```python
from build123d import *

# Parameters (mm, degrees)
SKETCH2_W               = 7
SKETCH2_H               = 2.5
REVOLVE2_ANGLE          = 180
BOSS_EXTRUDE4_DEPTH     = 24
CUT_EXTRUDE1_DEPTH      = 3.5
SKETCH17_W              = 3
SKETCH17_H              = 5
CUT_EXTRUDE6_DEPTH      = 18
SKETCH16_R              = 1.52
CUT_EXTRUDE5_DEPTH      = 3.857492994
CUT_EXTRUDE5_DEPTH_BACK = 41.857492994
SKETCH19_R              = 2.02
CUT_EXTRUDE7_DEPTH      = 3
SKETCH20_R              = 2.02
CUT_EXTRUDE8_DEPTH      = 3
SKETCH21_R              = 15
CUT_EXTRUDE9_DEPTH      = 6.5
SKETCH22_R              = 5
BOSS_EXTRUDE6_DEPTH     = 6.5
SKETCH23_W              = 2
SKETCH23_H              = 3
SKETCH24_W              = 2
SKETCH24_H              = 3
SKETCH25_R              = 2
CUT_EXTRUDE11_DEPTH     = 20.5000001
SKETCH26_R              = 3.17
CUT_EXTRUDE12_DEPTH     = 6.5


with BuildPart() as part:
    # Sketch1 → Revolve1 (revolve)
    with BuildSketch(Plane.XY):
        Polygon((0, 0), (12, 10), (17, 10), (22, 10), (22, 8), (19, 8), (19, -7), (0, -7), align=None)
    revolve(axis=Axis((0, -7, 0), (0, 1, 0)))

    # Sketch2 → Revolve2 (revolve)
    with BuildSketch(Plane(origin=(0, 10, 0), x_dir=(1, 0, 0), z_dir=(0, 1, 0))):
        with Locations((15.5, 1.25)):
            Rectangle(SKETCH2_W, SKETCH2_H)
        with Locations((-15.5, 1.25)):
            Rectangle(SKETCH2_W, SKETCH2_H)
    revolve(axis=Axis((0, 10, 0), (1, 0, 0)), revolution_arc=REVOLVE2_ANGLE)

    # Sketch8 → Boss-Extrude4 (add)
    with BuildSketch(Plane(origin=(-12, 0, 0), x_dir=(0, 0, -1), z_dir=(1, 0, 0))):
        with BuildLine():
            Line((-2.5, 10), (0, 10))
            Line((0, 10), (2.5, 10))
            ThreePointArc((2.5, 10), (0, 12.5), (-2.5, 10))
        make_face()
    extrude(amount=BOSS_EXTRUDE4_DEPTH)

    # Sketch9 → Cut-Extrude1 (cut, through all)
    with BuildSketch(Plane(origin=(0, 10, 0), x_dir=(1, 0, 0), z_dir=(0, 1, 0))):
        with BuildLine():
            ThreePointArc((-11.736694594, 2.5), (-12, 0), (-11.736694594, -2.5))
            ThreePointArc((-11.736694594, -2.5), (0, -12), (11.736694594, -2.5))
            ThreePointArc((11.736694594, -2.5), (12, 0), (11.736694594, 2.5))
            ThreePointArc((11.736694594, 2.5), (0, 12), (-11.736694594, 2.5))
        make_face()
    extrude(amount=CUT_EXTRUDE1_DEPTH, mode=Mode.SUBTRACT)

    # Sketch17 → Cut-Extrude6 (cut, through all)
    with BuildSketch(Plane(origin=(0, 10, 0), x_dir=(1, 0, 0), z_dir=(0, 1, 0))):
        with Locations((20.5, 0)):
            Rectangle(SKETCH17_W, SKETCH17_H)
        with Locations((-20.5, 0)):
            Rectangle(SKETCH17_W, SKETCH17_H)
    extrude(amount=-CUT_EXTRUDE6_DEPTH, mode=Mode.SUBTRACT)

    # Sketch16 → Cut-Extrude5 (cut, two sides)
    with BuildSketch(Plane.ZY.offset(19)) as cut_extrude5_sk:
        with Locations((0, 10)):
            Circle(SKETCH16_R)
    extrude(amount=CUT_EXTRUDE5_DEPTH, mode=Mode.SUBTRACT)
    extrude(cut_extrude5_sk.sketch, amount=-CUT_EXTRUDE5_DEPTH_BACK, mode=Mode.SUBTRACT)

    # Sketch19 → Cut-Extrude7 (cut)
    with BuildSketch(Plane.ZY.offset(19)):
        with Locations((0, 10)):
            Circle(SKETCH19_R)
    extrude(amount=-CUT_EXTRUDE7_DEPTH, mode=Mode.SUBTRACT)

    # Sketch20 → Cut-Extrude8 (cut)
    with BuildSketch(Plane(origin=(19, 0, 0), x_dir=(0, 0, -1), z_dir=(1, 0, 0))):
        with Locations((0, 10)):
            Circle(SKETCH20_R)
    extrude(amount=-CUT_EXTRUDE8_DEPTH, mode=Mode.SUBTRACT)

    # Sketch21 → Cut-Extrude9 (cut)
    with BuildSketch(Plane.XZ.offset(7)):
        Circle(SKETCH21_R)
    extrude(amount=-CUT_EXTRUDE9_DEPTH, mode=Mode.SUBTRACT)

    # Sketch22 → Boss-Extrude6 (add)
    with BuildSketch(Plane.XZ.offset(0.5)):
        Circle(SKETCH22_R)
    extrude(amount=BOSS_EXTRUDE6_DEPTH)

    # Cut-Sweep2: sweep along a curve in space
    with BuildLine() as cut_sweep2_path:
        Line((10, -0.5, 0), (16, 8.48, 0))
        Line((16, 8.48, 0), (16.813206723, 9.697099395, 0))
    # Sketch23 → Cut-Sweep2 (sweep, cut)
    with BuildSketch(Plane.XZ.offset(0.5)):
        with Locations((11, 0)):
            Rectangle(SKETCH23_W, SKETCH23_H)
    sweep(path=cut_sweep2_path.line, mode=Mode.SUBTRACT)

    # Cut-Sweep3: sweep along a curve in space
    with BuildLine() as cut_sweep3_path:
        Line((-10, -0.5, 0), (-16, 8.48, 0))
        Line((-16, 8.48, 0), (-16.813206723, 9.697099395, 0))
    # Sketch24 → Cut-Sweep3 (sweep, cut)
    with BuildSketch(Plane.XZ.offset(0.5)):
        with Locations((-11, 0)):
            Rectangle(SKETCH24_W, SKETCH24_H)
    sweep(path=cut_sweep3_path.line, mode=Mode.SUBTRACT)

    # Sketch25 → Cut-Extrude11 (cut, through all)
    with BuildSketch(Plane.XZ.offset(7)):
        Circle(SKETCH25_R)
    extrude(amount=-CUT_EXTRUDE11_DEPTH, mode=Mode.SUBTRACT)

    # Sketch26 → Cut-Extrude12 (cut)
    with BuildSketch(Plane.XZ.offset(7)):
        Circle(SKETCH26_R)
    extrude(amount=-CUT_EXTRUDE12_DEPTH, mode=Mode.SUBTRACT)


solid = part.part
```
Can you work these out from the model? Positions are in its coordinate system, mm. A direction names the side the tool comes from. Coordinates: 2 decimals unless noted, no trailing zeros. Order: outer loops, then holes, each group sorted by start corner. A loop starts at its lowest first (then second) coordinate and runs counter-clockwise, first axis right, second up.
1. If we section it at C-C (y = 5.25): Please give me the cut outline in (x, z), then the cut area to 3 significant figures.
2. Thinking about a two-plate mould opening in Z: for faces 1 (the face through (1.5, 8, 19.1)), 2 (the face through (0, 9, -22)), 3 (the face through (-19, 12, 1)), which applies, +Z half, -Z half, draft (parallel to the pull), parting line (faces both ways), or undercut?
3. If we section it at A-A (x = 0): Please give me the cut outline in (y, z).
4. I need wall thicknesses on line 1 (Z direction, x = 0, y = -2.25); line 2 (Y direction, x = 18.4, z = 0); line 3 (Y direction, x = 14.1, z = 0). Which ranges of each line are inside material? Lowest first, please.
5. I'm going to push flat-ended pins straight in: pin 1 (15.5 mm diameter, centred on x = 10, z = -11, fed in from +Y); pin 2 (8 mm diameter, centred on y = 2.5, z = -15.5, fed in from -X); pin 3 (1.9 mm diameter, centred on x = 0.5, z = 1.5, fed in from -Y); pin 4 (4 mm diameter, centred on x = -3.5, z = 13, fed in from -Y). Where does each tip first touch, or does it pass through?
6. If we section it at D-D (x = -14): Please give me the cut outline in (y, z).
7. If we section it at B-B (z = 13.5): Please give me the cut outline in (x, y).
8. For faces 4 (the face through (17.521, 12.003, 0.263)), 5 (the face through (20, 9, -2.5)), 6 (the face through (14, 4, -1.5)), 7 (the face through (1.5, 8, -19.2)), 8 (the face through (-2.516, -3.796, -1.929)), which set-ups out of +Z, -Z, +X, -X, +Y, -Y let a thin tool reach every point of the face, with its end or its side?
Entries:
1. outline: circle Ø38 at (0, 0); hole (-15.84, -1.5) - (-13.84, -1.5) - (-13.84, 1.5) - (-15.84, 1.5) - close; hole circle Ø12.6 at (0, 0); hole (13.84, -1.5) - (15.84, -1.5) - (15.84, 1.5) - (13.84, 1.5) - close
1. area: 997 mm2
2. face 1: draft
2. face 2: -Z half
2. face 3: undercut
3. outline: (-7, -19) - (8, -19) - (8, -22) - (10, -22) - (10, -12) - (1.67, -2) - (-0.5, -2) - (-0.5, -3.17) - (-7, -3.17) - (-7, -5) - (-0.5, -5) - (-0.5, -15) - (-7, -15) - close; (-7, 3.17) - (-0.5, 3.17) - (-0.5, 2) - (1.67, 2) - (10, 12) - (10, 22) - (8, 22) - (8, 19) - (-7, 19) - (-7, 15) - (-0.5, 15) - (-0.5, 5) - (-7, 5) - close
4. line 1: z = -19 to -15, -5 to -3.17, 3.17 to 5, 15 to 19
4. line 2: y = -7 to 7.98, 12.02 to 12.5
4. line 3: y = -0.5 to 2.64, 5.64 to 8.48, 11.52 to 12.5
5. pin 1: stops at y = 10
5. pin 2: stops at x = -15.12
5. pin 3: stops at y = -0.5
5. pin 4: stops at y = -7
6. outline: (-7, -12.85) - (8, -12.85) - (8, -16.97) - (10, -16.97) - (10, -2.5) arc R2.5 ccw to (10, 2.5) - (10, 16.97) - (8, 16.97) - (8, 12.85) - (-7, 12.85) - (-7, 5.39) - (-0.5, 5.39) - (-0.5, -5.39) - (-7, -5.39) - close; hole (2.49, -1.5) - (5.49, -1.5) - (5.49, 1.5) - (2.49, 1.5) - close; hole circle Ø3.04 at (10, 0)
7. outline: (-17.37, 8) - (-13.37, 8) - (-13.37, -7) - (-6.54, -7) - (-6.54, -0.5) - (6.54, -0.5) - (6.54, -7) - (13.37, -7) - (13.37, 8) - (17.37, 8) - (17.37, 10) - (-17.37, 10) - close
8. face 4: +X
8. face 5: +X, +Y, -Y
8. face 6: none
8. face 7: -Z, -Y
8. face 8: -Y
